Geometry: see drawing. Coordinates: mm, zero at the bounding-box minimum. Coordinates: 2 decimals unless noted, no trailing zeros. Write each loop counter-clockwise with the first axis right and the second up, starting at its lowest first coordinate (ties: lowest second). Pieces come first, ordered by that corner, then holes. Notation, with made-up numbers: (8.25, -39) - (32.25, -39) arc R22 ccw to (32.25, -11) - close; hole circle Ø8 at (22.25, -38.5). An arc over 180 degrees is marked (long way). One line per question, with ' | ' between items. Start each with the question number.
Q1. Cut plane A-A, the plane x = 53. Return loops of the section in (y, z).
Q2. Contact query for a flat-ended pin moving along its axis: P1, Ø2, axis at x = 93.5, y = 1.5, coming from the +Z side. Output: stop coordinate, or through.
Q3. Line query: line 1 (Z direction, x = 74.5, y = 2.25) (1 decimal); line 2 (Z direction, x = 14, y = 4.5) (1 decimal); line 3 (Y direction, x = 29.5, z = 59). Output: solid intervals per line, ascending.
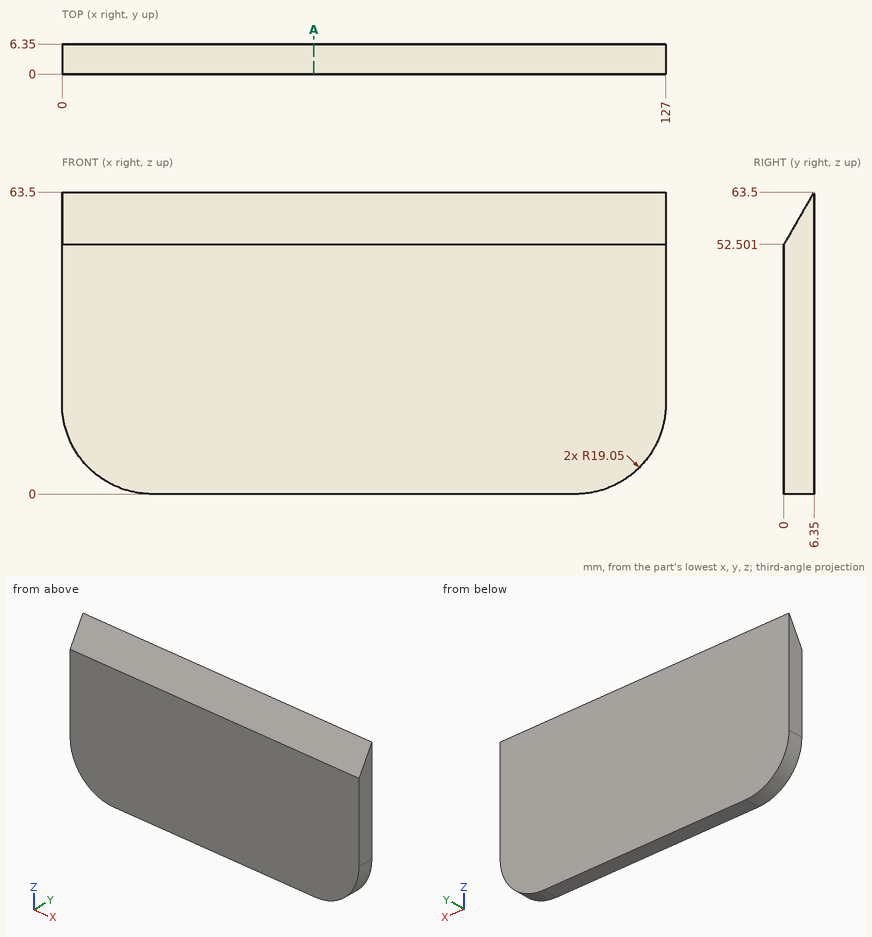
Reply:
1) outline: (0, 0) - (6.35, 0) - (6.35, 63.5) - (0, 52.5) - close
2) P1: stops at z = 56.83
3) line 1: z = 0 to 56.4 | line 2: z = 0.7 to 60.3 | line 3: y = 3.75 to 6.35
